from build123d import *

# Parameters (mm, degrees)
F0_W      = 28.8499742746
F0_H      = 37.8827601671
F1_DEPTH  = 16
F2_DEPTH  = 296
F3_DEPTH  = 996
F4_W      = 199.8313069344
F4_H      = 801.1276721954
F5_DEPTH  = 5
F6_DEPTH  = 39.21
F7_DEPTH  = 2.24
F8_DEPTH  = 55.66
F9_DEPTH  = 1.59
F10_W     = 54.77245152
F10_H     = 895.9976721954
F11_DEPTH = 5
F12_DEPTH = 5.86
F13_DEPTH = 18.91
F14_W     = 83.0026693535
F14_H     = 34.9487662315
F14_H_2   = 55.274695158
F15_W     = 82.9961860609
F15_H     = 44.8832511902
F15_H_2   = 52.5203943253
F16_DEPTH = 5
F17_DEPTH = 300
F18_DEPTH = 300
F19_DEPTH = 324.79
F20_DEPTH = 324.79
F21_DEPTH = 250
F22_DEPTH = 250
F23_DEPTH = 100
F24_DEPTH = 100
F25_DEPTH = 50
F26_DEPTH = 50
F27_DEPTH = 134.02
F28_DEPTH = 100
F29_DEPTH = 100
F30_DEPTH = 100
F31_DEPTH = 50
F32_DEPTH = 54.95
F33_DEPTH = 50
F34_DEPTH = 109.29
F35_DEPTH = 14.88
F36_DEPTH = 230.15
F37_DEPTH = 230.15
F38_DEPTH = 22.52
F39_DEPTH = 77.2
F40_DEPTH = 77.2
F41_DEPTH = 11
F42_DEPTH = 200
F43_DEPTH = 200
F44_DEPTH = 200
F45_DEPTH = 70
F46_DEPTH = 70
F47_DEPTH = 70
F48_DEPTH = 70
F49_DEPTH = 100
F50_DEPTH = 50
F51_DEPTH = 100
F52_DEPTH = 50
F53_R     = 3


with BuildPart() as f1:
    # F0 (on Front) → F1 (new body)
    with BuildSketch(Plane.XZ):
        with Locations((14.4249871373, 18.9413800836)):
            Rectangle(F0_W, F0_H)
    extrude(amount=F1_DEPTH)

    # F2 (add): a face of the model
    f2_faces = [f1.faces().sort_by_distance(p)[0] for p in [
        (0, -8, 18.9413800836),
    ]]
    extrude(f2_faces, amount=-F2_DEPTH)

    # F3 (add): a face of the model
    f3_faces = [f1.faces().sort_by_distance(p)[0] for p in [
        (148, -8, 0),
    ]]
    extrude(f3_faces, amount=-F3_DEPTH)

    # F4 (on face) → F5 (cut)
    with BuildSketch(Plane.XZ.offset(16)):
        with Locations((148.3252942562, 506.2239170074)):
            Rectangle(F4_W, F4_H)
    extrude(amount=-F5_DEPTH, mode=Mode.SUBTRACT)

    # F6 (cut): a face of the model
    f6_faces = [f1.faces().sort_by_distance(p)[0] for p in [
        (148.3252942562, -13.5, 906.7877531052),
    ]]
    extrude(f6_faces, amount=-F6_DEPTH, mode=Mode.SUBTRACT)

    # F7 (add): a face of the model
    f7_faces = [f1.faces().sort_by_distance(p)[0] for p in [
        (248.2409477234, -13.5, 525.8289170074),
    ]]
    extrude(f7_faces, amount=F7_DEPTH)

    # F8 (cut): a face of the model
    f8_faces = [f1.faces().sort_by_distance(p)[0] for p in [
        (147.2052942562, -13.5, 105.6600809097),
    ]]
    extrude(f8_faces, amount=-F8_DEPTH, mode=Mode.SUBTRACT)

    # F9 (add): a face of the model
    f9_faces = [f1.faces().sort_by_distance(p)[0] for p in [
        (48.409640789, -13.5, 497.9989170074),
    ]]
    extrude(f9_faces, amount=F9_DEPTH)

    # F10 (on face) → F11 (join)
    with BuildSketch(Plane.XZ.offset(11)):
        with Locations((154.5285359025, 497.9989170074)):
            Rectangle(F10_W, F10_H)
    extrude(amount=F11_DEPTH)

    # F12 (cut): a face of the model
    f12_faces = [f1.faces().sort_by_distance(p)[0] for p in [
        (127.1423101425, -13.5, 497.9989170074),
    ]]
    extrude(f12_faces, amount=-F12_DEPTH, mode=Mode.SUBTRACT)

    # F13 (cut): a face of the model
    f13_faces = [f1.faces().sort_by_distance(p)[0] for p in [
        (181.9147616625, -13.5, 497.9989170074),
    ]]
    extrude(f13_faces, amount=-F13_DEPTH, mode=Mode.SUBTRACT)

    # F14 (on face) + F15 (on face) → F16 (join)
    with BuildSketch(Plane.XZ.offset(11)):
        with Locations((91.5009754658, 853.3093035221)):
            Rectangle(F14_W, F14_H)
        with Locations((91.5009754658, 511.6568356752)):
            Rectangle(F14_W, F14_H_2)
    with BuildSketch(Plane.XZ.offset(11)):
        with Locations((204.5028546929, 853.7013530731)):
            Rectangle(F15_W, F15_H)
        with Locations((204.5028546929, 576.5425562859)):
            Rectangle(F15_W, F15_H_2)
    extrude(amount=F16_DEPTH)

    # F17 (add): faces of the model
    f17_faces = [f1.faces().sort_by_distance(p)[0] for p in [
        (204.5028546929, -13.5, 550.2823591232),
        (91.5009754658, -13.5, 484.0194880962),
    ]]
    extrude(f17_faces, amount=F17_DEPTH)

    # F18 (cut): faces of the model
    f18_faces = [f1.faces().sort_by_distance(p)[0] for p in [
        (91.5009754658, -13.5, 539.2941832542),
        (204.5028546929, -13.5, 602.8027534485),
    ]]
    extrude(f18_faces, amount=-F18_DEPTH, mode=Mode.SUBTRACT)

    # F19 (add): a face of the model
    f19_faces = [f1.faces().sort_by_distance(p)[0] for p in [
        (91.5009754658, -13.5, 835.8349204063),
    ]]
    extrude(f19_faces, amount=F19_DEPTH)

    # F20 (cut): a face of the model
    f20_faces = [f1.faces().sort_by_distance(p)[0] for p in [
        (91.5009754658, -13.5, 870.7836866379),
    ]]
    extrude(f20_faces, amount=-F20_DEPTH, mode=Mode.SUBTRACT)

    # F21 (add): a face of the model
    f21_faces = [f1.faces().sort_by_distance(p)[0] for p in [
        (91.5009754658, -13.5, 239.2941832542),
    ]]
    extrude(f21_faces, amount=F21_DEPTH)

    # F22 (cut): a face of the model
    f22_faces = [f1.faces().sort_by_distance(p)[0] for p in [
        (91.5009754658, -13.5, 184.0194880962),
    ]]
    extrude(f22_faces, amount=-F22_DEPTH, mode=Mode.SUBTRACT)

    # F23 (add): a face of the model
    f23_faces = [f1.faces().sort_by_distance(p)[0] for p in [
        (91.5009754658, -13.5, 545.9936866379),
    ]]
    extrude(f23_faces, amount=F23_DEPTH)

    # F24 (cut): a face of the model
    f24_faces = [f1.faces().sort_by_distance(p)[0] for p in [
        (91.5009754658, -13.5, 511.0449204063),
    ]]
    extrude(f24_faces, amount=-F24_DEPTH, mode=Mode.SUBTRACT)

    # F25 (add): a face of the model
    f25_faces = [f1.faces().sort_by_distance(p)[0] for p in [
        (91.5009754658, -13.5, 645.9936866379),
    ]]
    extrude(f25_faces, amount=F25_DEPTH)

    # F26 (cut): a face of the model
    f26_faces = [f1.faces().sort_by_distance(p)[0] for p in [
        (91.5009754658, -13.5, 611.0449204063),
    ]]
    extrude(f26_faces, amount=-F26_DEPTH, mode=Mode.SUBTRACT)

    # F27 (add): a face of the model
    f27_faces = [f1.faces().sort_by_distance(p)[0] for p in [
        (91.5009754658, -13.5, 434.0194880962),
    ]]
    extrude(f27_faces, amount=F27_DEPTH)

    # F28 (cut): a face of the model
    f28_faces = [f1.faces().sort_by_distance(p)[0] for p in [
        (91.5009754658, -13.5, 299.9994880962),
    ]]
    extrude(f28_faces, amount=-F28_DEPTH, mode=Mode.SUBTRACT)

    # F29 (add): a face of the model
    f29_faces = [f1.faces().sort_by_distance(p)[0] for p in [
        (91.5009754658, -13.5, 661.0449204063),
    ]]
    extrude(f29_faces, amount=F29_DEPTH)

    # F30 (cut): a face of the model
    f30_faces = [f1.faces().sort_by_distance(p)[0] for p in [
        (91.5009754658, -13.5, 695.9936866379),
    ]]
    extrude(f30_faces, amount=-F30_DEPTH, mode=Mode.SUBTRACT)

    # F31 (add): a face of the model
    f31_faces = [f1.faces().sort_by_distance(p)[0] for p in [
        (91.5009754658, -13.5, 595.9936866379),
    ]]
    extrude(f31_faces, amount=F31_DEPTH)

    # F32 (cut): a face of the model
    f32_faces = [f1.faces().sort_by_distance(p)[0] for p in [
        (91.5009754658, -13.5, 561.0449204063),
    ]]
    extrude(f32_faces, amount=-F32_DEPTH, mode=Mode.SUBTRACT)

    # F33 (add): a face of the model
    f33_faces = [f1.faces().sort_by_distance(p)[0] for p in [
        (91.5009754658, -13.5, 399.9994880962),
    ]]
    extrude(f33_faces, amount=F33_DEPTH)

    # F34 (cut): a face of the model
    f34_faces = [f1.faces().sort_by_distance(p)[0] for p in [
        (91.5009754658, -13.5, 489.2941832542),
    ]]
    extrude(f34_faces, amount=-F34_DEPTH, mode=Mode.SUBTRACT)

    # F35 (cut): a face of the model
    f35_faces = [f1.faces().sort_by_distance(p)[0] for p in [
        (204.5028546929, -13.5, 831.259727478),
    ]]
    extrude(f35_faces, amount=-F35_DEPTH, mode=Mode.SUBTRACT)

    # F36 (add): a face of the model
    f36_faces = [f1.faces().sort_by_distance(p)[0] for p in [
        (204.5028546929, -13.5, 846.139727478),
    ]]
    extrude(f36_faces, amount=F36_DEPTH)

    # F37 (cut): a face of the model
    f37_faces = [f1.faces().sort_by_distance(p)[0] for p in [
        (204.5028546929, -13.5, 876.1429786682),
    ]]
    extrude(f37_faces, amount=-F37_DEPTH, mode=Mode.SUBTRACT)

    # F38 (cut): a face of the model
    f38_faces = [f1.faces().sort_by_distance(p)[0] for p in [
        (204.5028546929, -13.5, 250.2823591232),
    ]]
    extrude(f38_faces, amount=-F38_DEPTH, mode=Mode.SUBTRACT)

    # F39 (add): a face of the model
    f39_faces = [f1.faces().sort_by_distance(p)[0] for p in [
        (204.5028546929, -13.5, 302.8027534485),
    ]]
    extrude(f39_faces, amount=F39_DEPTH)

    # F40 (cut): a face of the model
    f40_faces = [f1.faces().sort_by_distance(p)[0] for p in [
        (204.5028546929, -13.5, 272.8023591232),
    ]]
    extrude(f40_faces, amount=-F40_DEPTH, mode=Mode.SUBTRACT)

    # F41 (cut): faces of the model
    f41_faces = [f1.faces().sort_by_distance(p)[0] for p in [
        (91.5009754658, -11, 795.9957198715),
        (204.5028546929, -11, 795.9953658867),
        (204.5028546929, -11, 497.9962404633),
        (91.5009754658, -11, 497.9995518303),
        (91.5009754658, -11, 199.999784503),
        (204.5028546929, -11, 200.0012200165),
    ]]
    extrude(f41_faces, amount=-F41_DEPTH, mode=Mode.SUBTRACT)

    # F42 (add): faces of the model
    f42_faces = [f1.faces().sort_by_distance(p)[0] for p in [
        (204.5028546929, -8, 615.989727478),
        (91.5009754658, -8, 615.9949204063),
    ]]
    extrude(f42_faces, amount=F42_DEPTH)

    # F43 (add): faces of the model
    f43_faces = [f1.faces().sort_by_distance(p)[0] for p in [
        (91.5009754658, -8, 945.9977531052),
        (204.5028546929, -8, 945.9977531052),
    ]]
    extrude(f43_faces, amount=F43_DEPTH)

    # F44 (cut): faces of the model
    f44_faces = [f1.faces().sort_by_distance(p)[0] for p in [
        (148, -8, 996),
        (91.5009754658, -8, 645.9936866379),
        (204.5028546929, -8, 645.9929786682),
    ]]
    extrude(f44_faces, amount=-F44_DEPTH, mode=Mode.SUBTRACT)

    # F45 (add): faces of the model
    f45_faces = [f1.faces().sort_by_distance(p)[0] for p in [
        (204.5028546929, -8, 350.0023591232),
        (91.5009754658, -8, 349.9994880962),
    ]]
    extrude(f45_faces, amount=F45_DEPTH)

    # F46 (cut): faces of the model
    f46_faces = [f1.faces().sort_by_distance(p)[0] for p in [
        (204.5028546929, -8, 380.0027534485),
        (91.5009754658, -8, 380.0041832542),
    ]]
    extrude(f46_faces, amount=-F46_DEPTH, mode=Mode.SUBTRACT)

    # F47 (add): faces of the model
    f47_faces = [f1.faces().sort_by_distance(p)[0] for p in [
        (204.5028546929, -8, 445.9929786682),
        (91.5009754658, -8, 445.9936866379),
    ]]
    extrude(f47_faces, amount=F47_DEPTH)

    # F48 (cut): faces of the model
    f48_faces = [f1.faces().sort_by_distance(p)[0] for p in [
        (204.5028546929, -8, 415.989727478),
        (91.5009754658, -8, 415.9949204063),
    ]]
    extrude(f48_faces, amount=-F48_DEPTH, mode=Mode.SUBTRACT)

    # F49 (add): a face of the model
    f49_faces = [f1.faces().sort_by_distance(p)[0] for p in [
        (296, -8, 398),
    ]]
    extrude(f49_faces, amount=F49_DEPTH)

    # F50 (add): faces of the model
    f50_faces = [f1.faces().sort_by_distance(p)[0] for p in [
        (163.0047616625, -8, 397.9962404633),
        (163.0047616625, -8, 165.0012200165),
        (163.0047616625, -8, 630.9953658867),
    ]]
    extrude(f50_faces, amount=F50_DEPTH)

    # F51 (cut): faces of the model
    f51_faces = [f1.faces().sort_by_distance(p)[0] for p in [
        (246.0009477234, -8, 630.9953658867),
        (246.0009477234, -8, 397.9962404633),
        (246.0009477234, -8, 165.0012200165),
    ]]
    extrude(f51_faces, amount=-F51_DEPTH, mode=Mode.SUBTRACT)

    # F52 (cut): faces of the model
    f52_faces = [f1.faces().sort_by_distance(p)[0] for p in [
        (133.0023101425, -8, 397.9995518303),
        (133.0023101425, -8, 630.9957198715),
        (133.0023101425, -8, 164.999784503),
    ]]
    extrude(f52_faces, amount=-F52_DEPTH, mode=Mode.SUBTRACT)

    # F53
    f53_edges = [f1.edges().sort_by_distance(p)[0] for p in [
        (0, -16, 398),
        (198, -16, 0),
        (396, -16, 398),
        (198, -16, 796),
        (116.500975, -16, 279.999488),
        (183.00231, -16, 164.999785),
        (116.500975, -16, 50.000081),
        (49.999641, -16, 164.999785),
        (279.502855, -16, 280.002359),
        (346.000948, -16, 165.00122),
        (279.502855, -16, 50.000081),
        (213.004762, -16, 165.00122),
        (279.502855, -16, 310.002753),
        (213.004762, -16, 397.99624),
        (279.502855, -16, 485.989727),
        (346.000948, -16, 397.99624),
        (116.500975, -16, 310.004183),
        (49.999641, -16, 397.999552),
        (116.500975, -16, 485.99492),
        (183.00231, -16, 397.999552),
        (116.500975, -16, 515.993687),
        (49.999641, -16, 630.99572),
        (116.500975, -16, 745.997753),
        (183.00231, -16, 630.99572),
        (213.004762, -16, 630.995366),
        (279.502855, -16, 745.997753),
        (346.000948, -16, 630.995366),
        (279.502855, -16, 515.992979),
    ]]
    fillet(f53_edges, radius=F53_R)


solid = f1.part
Design review of the part built by this model. Coordinates are the model's own, in mm. Give positions to 0.01 mm unless a question says otherwise; leave off trailing zeros. Loops run counter-clockwise (first coordinate to the right, second up) from the corner with the lowest first, then second, coordinate; pieces in that order, holes last. Notation, with made-up numbers: M 88,-33 L 106,-33 A20 ccw 106,-10 Z; hole C -4,-35 d5. An arc over 180 degrees is marked long. Write item = value, one per line.
Q1. To check wall thickness, follow line 1 (X direction, y = -11, z = 235); line 2 (Z direction, x = 237, y = -5); line 3 (X direction, y = -14, z = 409). State the ranges of each line that lie inside material, in increasing order. Write a range as [from, to].
Output values:
line_1 = [0, 50], [183, 213], [346, 396]
line_2 = [0, 50], [280, 310], [485.99, 515.99], [746, 796]
line_3 = [0.17, 49.83], [183.17, 212.83], [346.17, 395.83]
Q2. We need section A-A (x = 323). Give the boundary of the cut face in (y, z), plus the area to 3 significant figures.
Output values:
outline = M -16,3 A3 ccw -13,0 L 0,0 L 0,50 L -13,50 A3 ccw -16,47 Z; M -16,283 A3 ccw -13,280 L 0,280 L 0,310 L -13,310 A3 ccw -16,307 Z; M -16,488.99 A3 ccw -13,485.99 L 0,485.99 L 0,515.99 L -13,515.99 A3 ccw -16,512.99 Z; M -16,749 A3 ccw -13,746 L 0,746 L 0,796 L -13,796 A3 ccw -16,793 Z
area = 2,540 mm^2
Q3. We need section C-C (y = -6.5). Give the boundary of the cut face in (x, z).
Output values:
outline = M 0,0 L 396,0 L 396,796 L 0,796 Z; hole M 50,50 L 183,50 L 183,280 L 50,280 Z; hole M 50,310 L 183,310 L 183,485.99 L 50,485.99 Z; hole M 50,515.99 L 183,515.99 L 183,746 L 50,746 Z; hole M 213,50 L 346,50 L 346,280 L 213,280 Z; hole M 213,310 L 346,310 L 346,485.99 L 213,485.99 Z; hole M 213,515.99 L 346,515.99 L 346,746 L 213,746 Z
Q4. We need section B-B (z = 218). Give the boundary of the cut face in (x, y).
Output values:
outline = M 0,-13 A3 ccw 3,-16 L 47,-16 A3 ccw 50,-13 L 50,0 L 0,0 Z; M 183,-13 A3 ccw 186,-16 L 210,-16 A3 ccw 213,-13 L 213,0 L 183,0 Z; M 346,-13 A3 ccw 349,-16 L 393,-16 A3 ccw 396,-13 L 396,0 L 346,0 Z
